```python
from build123d import *

# Parameters (mm, degrees)
SKETCH_1_R          = 1.25
EXTRUDE_1_DEPTH     = 5
SKETCH_2_R          = 1
EXTRUDE_8_DEPTH     = 4
EXTRUDE_START       = -2
SKETCH_2_2_R        = 1
EXTRUDE_9_DEPTH     = 2
EXTRUDE_10_DEPTH    = 2
CUT_EXTRUDE_START   = -0.75
CUT_EXTRUDE_1_DEPTH = 0.75
FILLET_2_R          = 0.5


with BuildPart() as part:
    # Sketch 1 → Extrude 1 (new, symmetric)
    with BuildSketch(Plane(origin=(0, 0, 0), x_dir=(0, 0, -1), z_dir=(1, 0, 0))):
        with BuildLine():
            Line((-1.75, 2.202634141), (1.75, 2.202634141))
            Line((1.75, 2.202634141), (1.75, -0.028893504))
            ThreePointArc((1.75, -0.028893504), (0, -1.797365859), (-1.75, -0.028893504))
            Line((-1.75, -0.028893504), (-1.75, 2.202634141))
        make_face()
        with Locations((0, -0.047269384)):
            Circle(SKETCH_1_R, mode=Mode.SUBTRACT)
    extrude(amount=EXTRUDE_1_DEPTH, both=True)

    # Sketch 2 → Extrude 8 (add)
    with BuildSketch(Plane(origin=(0, 2.202634141, 0), x_dir=(1, 0, 0), z_dir=(0, 1, 0))):
        with Locations(Location((3, 0, 0), (0, 0, 90))):
            Circle(SKETCH_2_R)
        with Locations(Location((-3, 0, 0), (0, 0, 90))):
            Circle(SKETCH_2_R)
    extrude(amount=EXTRUDE_8_DEPTH)

    # Sketch 2_2 → Extrude 9 (add)
    with BuildSketch(Plane(origin=(0, 2.202634141, 0), x_dir=(1, 0, 0), z_dir=(0, 1, 0)).offset(EXTRUDE_START)):
        with Locations(Location((3, 0, 0), (0, 0, 90))):
            Circle(SKETCH_2_2_R)
        with Locations(Location((-3, 0, 0), (0, 0, 90))):
            Circle(SKETCH_2_2_R)
    extrude(amount=EXTRUDE_9_DEPTH)

    # Sketch 4 → Extrude 10 (add)
    with BuildSketch(Plane(origin=(0, 6.202634141, 0), x_dir=(1, 0, 0), z_dir=(0, 1, 0)).offset(EXTRUDE_START)):
        with BuildLine():
            Line((-3.38295337, 0.923767674), (-4.212535059, 1.590521528))
            ThreePointArc((-4.212535059, 1.590521528), (-4.571679225, 1.236860709), (-4.830997986, 0.804640526))
            Line((-4.830997986, 0.804640526), (-3.991522536, 0.12993483))
            ThreePointArc((-3.991522536, 0.12993483), (-3.793623746, 0.608408867), (-3.38295337, 0.923767674))
        make_face()
        with BuildLine():
            Line((-1.185902953, -0.842052198), (-2.015484642, -0.175298344))
            ThreePointArc((-2.015484642, -0.175298344), (-2.235131848, -0.64418686), (-2.659841227, -0.940368018))
            Line((-2.659841227, -0.940368018), (-1.820365778, -1.615073714))
            ThreePointArc((-1.820365778, -1.615073714), (-1.454038392, -1.26885882), (-1.185902953, -0.842052198))
        make_face()
        with BuildLine():
            Line((-3.991522536, 0.12993483), (-4.830997986, 0.804640526))
            ThreePointArc((-4.830997986, 0.804640526), (-4.252925752, -1.558902518), (-1.820365778, -1.615073714))
            Line((-1.820365778, -1.615073714), (-2.659841227, -0.940368018))
            ThreePointArc((-2.659841227, -0.940368018), (-3.626462876, -0.779451259), (-3.991522536, 0.12993483))
        make_face()
        with BuildLine():
            ThreePointArc((-1, 0), (-2.112607786, 1.792354613), (-4.212535059, 1.590521528))
            Line((-4.212535059, 1.590521528), (-3.38295337, 0.923767674))
            ThreePointArc((-3.38295337, 0.923767674), (-2.444551249, 0.831550771), (-2, 0))
            ThreePointArc((-2, 0), (-2.003878683, -0.087990459), (-2.015484642, -0.175298344))
            Line((-2.015484642, -0.175298344), (-1.185902953, -0.842052198))
            ThreePointArc((-1.185902953, -0.842052198), (-1.047028662, -0.431164647), (-1, 0))
        make_face()
        with BuildLine():
            ThreePointArc((-2, 0), (-2.444551249, 0.831550771), (-3.38295337, 0.923767674))
            Line((-3.38295337, 0.923767674), (-2.015484642, -0.175298344))
            ThreePointArc((-2.015484642, -0.175298344), (-2.003878683, -0.087990459), (-2, 0))
        make_face()
        with BuildLine():
            Line((-2.015484642, -0.175298344), (-3.38295337, 0.923767674))
            ThreePointArc((-3.38295337, 0.923767674), (-3.793623746, 0.608408867), (-3.991522536, 0.12993483))
            Line((-3.991522536, 0.12993483), (-2.659841227, -0.940368018))
            ThreePointArc((-2.659841227, -0.940368018), (-2.235131848, -0.64418686), (-2.015484642, -0.175298344))
        make_face()
        with BuildLine():
            Line((-2.659841227, -0.940368018), (-3.991522536, 0.12993483))
            ThreePointArc((-3.991522536, 0.12993483), (-3.626462876, -0.779451259), (-2.659841227, -0.940368018))
        make_face()
        with BuildLine():
            Line((1.185902953, -0.842052198), (4.212535059, 1.590521528))
            ThreePointArc((4.212535059, 1.590521528), (1.747074248, 1.558902518), (1.185902953, -0.842052198))
        make_face()
        with BuildLine():
            Line((1.820365778, -1.615073714), (4.830997986, 0.804640526))
            ThreePointArc((4.830997986, 0.804640526), (4.571679225, 1.236860709), (4.212535059, 1.590521528))
            Line((4.212535059, 1.590521528), (1.185902953, -0.842052198))
            ThreePointArc((1.185902953, -0.842052198), (1.454038392, -1.26885882), (1.820365778, -1.615073714))
        make_face()
        with BuildLine():
            ThreePointArc((5, 0), (4.957293536, 0.411098546), (4.830997986, 0.804640526))
            Line((4.830997986, 0.804640526), (1.820365778, -1.615073714))
            ThreePointArc((1.820365778, -1.615073714), (3.905740458, -1.783152888), (5, 0))
        make_face()
    extrude(amount=EXTRUDE_10_DEPTH)

    # Sketch 4_3 → Cut-Extrude 1 (cut)
    with BuildSketch(Plane(origin=(0, 6.202634141, 0), x_dir=(1, 0, 0), z_dir=(0, 1, 0)).offset(CUT_EXTRUDE_START)):
        with BuildLine():
            Line((-2.015484642, -0.175298344), (-3.38295337, 0.923767674))
            ThreePointArc((-3.38295337, 0.923767674), (-3.793623746, 0.608408867), (-3.991522536, 0.12993483))
            Line((-3.991522536, 0.12993483), (-2.659841227, -0.940368018))
            ThreePointArc((-2.659841227, -0.940368018), (-2.235131848, -0.64418686), (-2.015484642, -0.175298344))
        make_face()
        with BuildLine():
            Line((-3.38295337, 0.923767674), (-4.212535059, 1.590521528))
            ThreePointArc((-4.212535059, 1.590521528), (-4.571679225, 1.236860709), (-4.830997986, 0.804640526))
            Line((-4.830997986, 0.804640526), (-3.991522536, 0.12993483))
            ThreePointArc((-3.991522536, 0.12993483), (-3.793623746, 0.608408867), (-3.38295337, 0.923767674))
        make_face()
        with BuildLine():
            Line((-1.185902953, -0.842052198), (-2.015484642, -0.175298344))
            ThreePointArc((-2.015484642, -0.175298344), (-2.235131848, -0.64418686), (-2.659841227, -0.940368018))
            Line((-2.659841227, -0.940368018), (-1.820365778, -1.615073714))
            ThreePointArc((-1.820365778, -1.615073714), (-1.454038392, -1.26885882), (-1.185902953, -0.842052198))
        make_face()
        with BuildLine():
            Line((1.820365778, -1.615073714), (4.830997986, 0.804640526))
            ThreePointArc((4.830997986, 0.804640526), (4.571679225, 1.236860709), (4.212535059, 1.590521528))
            Line((4.212535059, 1.590521528), (1.185902953, -0.842052198))
            ThreePointArc((1.185902953, -0.842052198), (1.454038392, -1.26885882), (1.820365778, -1.615073714))
        make_face()
    extrude(amount=CUT_EXTRUDE_1_DEPTH, mode=Mode.SUBTRACT)

    # Fillet 2
    fillet_2_edges = [part.edges().sort_by_distance(p)[0] for p in [
        (-4.814097047, 4.202634141, -0.842052198),
        (4.179634222, 4.202634141, -1.615073714),
        (1.747074248, 6.202634141, -1.558902518),
        (4.252925752, 6.202634141, 1.558902518),
        (-1.747074248, 6.202634141, -1.558902518),
        (-4.252925752, 6.202634141, 1.558902518),
        (0, 2.202634141, 1.75),
        (0, 2.202634141, -1.75),
    ]]
    fillet(fillet_2_edges, radius=FILLET_2_R)


solid = part.part
```
Geometry check sheet. Reference: the model listing, model coordinates, mm. A direction names the side the tool comes from. Round coordinates to 2 decimals unless told otherwise and drop trailing zeros. Write each loop counter-clockwise with the first axis right and the second up, starting at its lowest first coordinate (ties: lowest second). Pieces come first, ordered by that corner, then holes. Notation, with made-up numbers: (26.5, 76) - (66.5, 76) arc R23 cw to (66.5, 108) - close; hole circle Ø8 at (76.5, 29). An arc over 180 degrees is marked (long way). Write each question's results on one line, items separated by ' | '.
(1) Set-up check for faces 1 (the face through (-3, 5.453, 0)), 2 (the face through (3, 0.203, 0)), 3 (the face through (3.6, 0.6, 0.8)): record each of +Z, -Z, +X, -X, +Y, -Y from which the full face is reachable in a straight line by a thin tool's end or side.
Computed:
face 1: +Y | face 2: +X, -X | face 3: none
(2) Thickness scan on probe 1 along Y at (x, z) = (1.5, 0); probe 2 along X at (y, z) = (3, 0.05); probe 3 along Y at (x, z) = (2.25, 1). Record the ranges inside material, lowest first. Write a range as from..to.
Computed:
probe 1: y = -1.8..-1.3, 1.2..2.2, 4.2..6.2 | probe 2: x = -4..-2, 2..4 | probe 3: y = -1.48..-0.8, 0.7..2.2, 4.2..5.45
(3) Sectioned sample at B-B, the plane x = 0.5. Enter the section's corners in (y, z), plus the area to 3 significant figures.
Computed:
outline: (-0.03, -1.75) - (1.7, -1.75) arc R0.5 ccw to (2.2, -1.25) - (2.2, 1.25) arc R0.5 ccw to (1.7, 1.75) - (-0.03, 1.75) arc R1.75 ccw (long way) to start; hole circle Ø2.5 at (-0.05, 0) | area: 7.67 mm^2
(4) Draft check along Y on faces 4 (the face through (0, 1, 1.75)), 5 (the face through (-0.07, -1.268, 0.271)), 6 (the face through (-3.6, 6.203, 0.7)). Enter one of: pulls with the +Y half, pulls with the -Y half, needs draft (parallel to the pull), parting line crosses it, or undercut.
Computed:
face 4: needs draft | face 5: undercut | face 6: pulls with the +Y half
(5) Sectioned sample at A-A, the plane y = 2.75. Enter the section's corners in (x, z), plus the area to 3 significant figures.
Computed:
outline: circle Ø2 at (-3, 0); circle Ø2 at (3, 0) | area: 6.28 mm^2
(6) Depth check by flat-ended pin: pin 1 Ø1 at (x, z) = (-2.5, 0.5) entering from +Y; pin 2 Ø1.5 at (y, z) = (-0.05, 0) entering from -X; pin 3 Ø1 at (x, y) = (4, 5) entering from -Z; pin 4 Ø3 at (x, y) = (3, 1) entering from +Z. Enter the tip coordinate at first touch or a pass-through.
Computed:
pin 1: stops at y = 6.2 | pin 2: stops at x = -4 | pin 3: stops at z = -1.94 | pin 4: stops at z = 1.75
